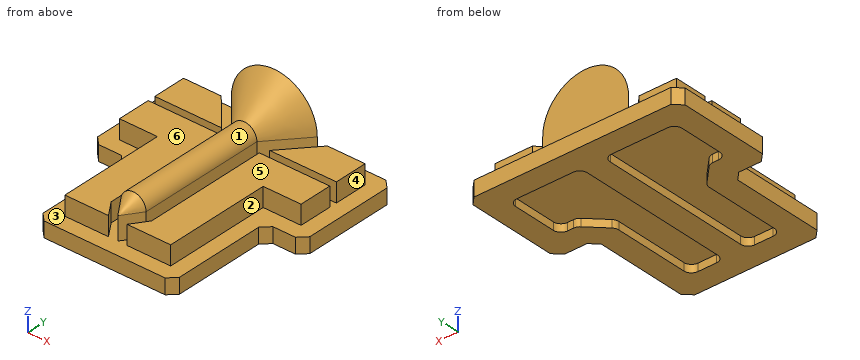
```python
from build123d import *

# Parameters (mm, degrees)
F1_DEPTH = 100
F2_DEPTH = 125
F3_DEPTH = 150
F5_ANGLE = 180
F6_SIZE  = 50
F8_DEPTH = 50
F9_R     = 50


with BuildPart() as f1:
    # F0 (on Top) → F1 (new body)
    with BuildSketch(Plane.XY):
        Polygon((694, 100), (0, 100), (-694, 100), (-694, -585.6), (-446, -585.6), (-446, -1286.9), (0, -1286.9), (446, -1286.9), (446, -585.6), (694, -585.6), align=None)
        Polygon((-594, -485.6), (-594, -267.8), (-132.6, -267.8), (-132.6, -1083.6631870207), (-60.8812384181, -1186.9), (-346, -1186.9), (-346, -485.6), align=None, mode=Mode.SUBTRACT)
        Polygon((132.6, -267.8), (594, -267.8), (594, -485.6), (346, -485.6), (346, -1186.9), (60.8812384181, -1186.9), (132.6, -1083.6631870207), align=None, mode=Mode.SUBTRACT)
        Polygon((-281.1, 0), (0, 0), (281.1, 0), (82.6, -227.7), (82.6, -1068), (0, -1186.9), (-82.6, -1068), (-82.6, -227.7), align=None, mode=Mode.SUBTRACT)
        Polygon((-594, -217.8), (-594, 0), (-347.4318814101, 0), (-157.5623161927, -217.8), align=None, mode=Mode.SUBTRACT)
        Polygon((594, -217.8), (157.5623161927, -217.8), (347.4318814101, 0), (594, 0), align=None, mode=Mode.SUBTRACT)
        Polygon((-347.4318814101, 0), (-594, 0), (-594, -217.8), (-157.5623161927, -217.8), align=None)
        Polygon((-132.6, -267.8), (-594, -267.8), (-594, -485.6), (-346, -485.6), (-346, -1186.9), (-60.8812384181, -1186.9), (-132.6, -1083.6631870207), align=None)
        Polygon((281.1, 0), (0, 0), (0, -1186.9), (82.6, -1068), (82.6, -227.7), align=None)
        Polygon((594, -485.6), (594, -267.8), (132.6, -267.8), (132.6, -1083.6631870207), (60.8812384181, -1186.9), (346, -1186.9), (346, -485.6), align=None)
        Polygon((347.4318814101, 0), (157.5623161927, -217.8), (594, -217.8), (594, 0), align=None)
        Polygon((0, -1186.9), (0, 0), (-281.1, 0), (-82.6, -227.7), (-82.6, -1068), align=None)
    extrude(amount=-F1_DEPTH)

    # F0 (on Top) → F2 (join)
    with BuildSketch(Plane.XY):
        Polygon((-347.4318814101, 0), (-594, 0), (-594, -217.8), (-157.5623161927, -217.8), align=None)
        Polygon((-132.6, -267.8), (-594, -267.8), (-594, -485.6), (-346, -485.6), (-346, -1186.9), (-60.8812384181, -1186.9), (-132.6, -1083.6631870207), align=None)
        Polygon((594, -485.6), (594, -267.8), (132.6, -267.8), (132.6, -1083.6631870207), (60.8812384181, -1186.9), (346, -1186.9), (346, -485.6), align=None)
        Polygon((347.4318814101, 0), (157.5623161927, -217.8), (594, -217.8), (594, 0), align=None)
    extrude(amount=F2_DEPTH)

    # F0 (on Top) → F3 (join)
    with BuildSketch(Plane.XY):
        Polygon((0, -1186.9), (0, 0), (-281.1, 0), (-82.6, -227.7), (-82.6, -1068), align=None)
        Polygon((281.1, 0), (0, 0), (0, -1186.9), (82.6, -1068), (82.6, -227.7), align=None)
    extrude(amount=F3_DEPTH)

    # F4 (on face) → F5 (revolve)
    with BuildSketch(Plane.XY.offset(150)):
        Polygon((0, -1186.9), (0, 0), (-281.1, 0), (-82.6, -227.7), (-82.6, -1068), align=None)
    revolve(axis=Axis((0, -593.45, 150), (0, 1, 0)), revolution_arc=F5_ANGLE)

    # F6
    f6_edges = [f1.edges().sort_by_distance(p)[0] for p in [
        (-694, 100, -50),
        (-694, -585.6, -50),
        (-446, -1286.9, -50),
        (446, -1286.9, -50),
        (-446, -585.6, -50),
        (446, -585.6, -50),
        (694, -585.6, -50),
        (694, 100, -50),
    ]]
    chamfer(f6_edges, length=F6_SIZE)

    # F7 (on face) → F8 (cut)
    with BuildSketch(Plane(origin=(0, 0, -100), x_dir=(1, 0, 0), z_dir=(0, 0, -1))):
        Polygon((-433.867965644, 435.6), (-544, 435.6), (-544, 50), (-75, 50), (-75, 1136.9), (-296, 1136.9), (-296, 573.467965644), align=None)
        Polygon((75, 1136.9), (75, 50), (544, 50), (544, 435.6), (433.867965644, 435.6), (296, 573.467965644), (296, 1136.9), align=None)
    extrude(amount=-F8_DEPTH, mode=Mode.SUBTRACT)

    # F9
    f9_edges = [f1.edges().sort_by_distance(p)[0] for p in [
        (-544, -435.6, -75),
        (-433.867966, -435.6, -75),
        (-296, -573.467966, -75),
        (-296, -1136.9, -75),
        (-75, -1136.9, -75),
        (-75, -50, -75),
        (-544, -50, -75),
        (75, -50, -75),
        (544, -50, -75),
        (544, -435.6, -75),
        (433.867966, -435.6, -75),
        (296, -573.467966, -75),
        (296, -1136.9, -75),
        (75, -1136.9, -75),
    ]]
    fillet(f9_edges, radius=F9_R)


solid = f1.part
```
Read the model definition and answer for the solid it produces. Units are mm, in the model's axes. Face numbers are marked on the shaded views. A direction names the side the tool comes from. Give positions to 0.01 mm unless a question says otherwise; leave off trailing zeros. Order: outer loops, then holes, each group sorted by start corner. A loop starts at its lowest first (then second) coordinate and runs counter-clockwise, first axis right, second up.
(1) For the marked faces 4, 5 and 6, determine the directions among +Z, -Z, +X, -X, +Y, -Y from which every point of the face is accessible in a straight line to the end or side of a thin tool.
(2) For a pull along X with two mould halves and no side action, classify the marked faces 1, 2 and 3 as released by +X, released by -X, zero draft, split by the parting line, or undercut.
(3) Find section C-C (y = -119.5). Give the vertices of the cut face in (x, z), plus the area to 3 significant figures.
(4) Find section B-B (x = -524.5). Give the vertices of the cut face in (y, z), plus the area to 3 significant figures.
(5) Find section A-A (y = -302). Give the vertices of the cut face in (x, z).
(6) Given pin 1 (5 mm diameter, centred on x = -234, z = 226.5, fed in from -Y); pin 2 (4 mm diameter, centred on x = 229.5, z = 304, fed in from -Y); pin 3 (3 mm diameter, centred on x = 88, z = 188.5, fed in from -Y), each flat-ended and moving along its own axis, determine where each tip first touches the part or whether it passes through.
(7) Straight lines are drawn through the part: L1, parallel to X at y = -1017, z = -72.5; L2, parallel to X at y = -314.5, z = 29.5; L3, parallel to Y at x = 503, z = 53. For each, find the intervals that lie inside material, in ascending order.
Result sheet:
1. face 4: +Z, +X, +Y, -Y
1. face 5: +Z, +X, -Y
1. face 6: +Z, -X, -Y
2. face 1: split by the parting line
2. face 2: released by +X
2. face 3: undercut
3. outline: (-694, -100) - (-544, -100) - (-544, -50) - (-75, -50) - (-75, -100) - (75, -100) - (75, -50) - (544, -50) - (544, -100) - (694, -100) - (694, 0) - (594, 0) - (594, 125) - (243.26, 125) - (243.26, 0) - (176.92, 0) - (176.92, 150) arc R176.92 ccw to (-176.92, 150) - (-176.92, 0) - (-243.26, 0) - (-243.26, 125) - (-594, 125) - (-594, 0) - (-694, 0) - close
3. area: 282,000 mm2
4. outline: (-585.6, -100) - (-425.22, -100) - (-425.22, -50) - (-60.38, -50) - (-60.38, -100) - (100, -100) - (100, 0) - (0, 0) - (0, 125) - (-217.8, 125) - (-217.8, 0) - (-267.8, 0) - (-267.8, 125) - (-485.6, 125) - (-485.6, 0) - (-585.6, 0) - close
4. area: 105,000 mm2
5. outline: (-694, -100) - (-544, -100) - (-544, -50) - (-75, -50) - (-75, -100) - (75, -100) - (75, -50) - (544, -50) - (544, -100) - (694, -100) - (694, 0) - (594, 0) - (594, 125) - (132.6, 125) - (132.6, 0) - (82.6, 0) - (82.6, 150) arc R82.6 ccw to (-82.6, 150) - (-82.6, 0) - (-132.6, 0) - (-132.6, 125) - (-594, 125) - (-594, 0) - (-694, 0) - close
6. pin 1: stops at y = -42.92
6. pin 2: stops at y = -7.71
6. pin 3: stops at y = -213.99
7. L1: x = -446 to -296, -75 to 75, 296 to 446
7. L2: x = -594 to -132.6, -82.6 to 82.6, 132.6 to 594
7. L3: y = -485.6 to -267.8, -217.8 to 0
